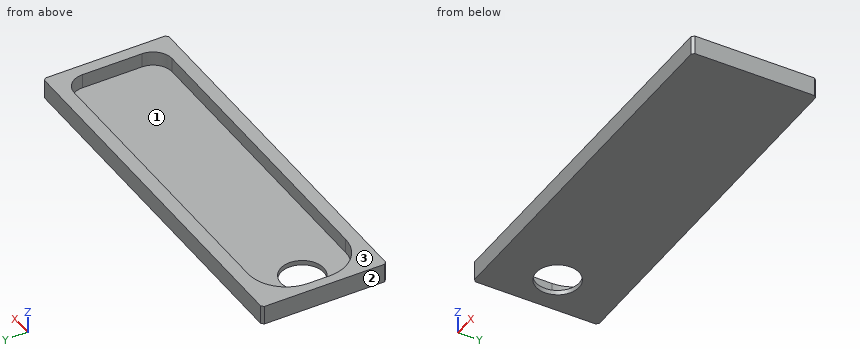
from build123d import *

# Parameters (mm, degrees)
F1_DEPTH = 3
F0_R     = 4.5
F2_DEPTH = 1
F3_SIZE  = 0.5


with BuildPart() as f1:
    # F0 (on Top) → F1 (new body)
    with BuildSketch(Plane.XY):
        Polygon((71.2, 13.05), (-8, 13.1), (-8, -13.1), (71.2, -13.05), align=None)
        with BuildLine():
            ThreePointArc((-6, 2.25), (-3.6568542495, 7.9068542495), (2, 10.25))
            Line((2, 10.25), (64.7, 10.25))
            ThreePointArc((64.7, 10.25), (67.5284271247, 9.0784271247), (68.7, 6.25))
            Line((68.7, 6.25), (68.7, -6.25))
            ThreePointArc((68.7, -6.25), (67.5284271247, -9.0784271247), (64.7, -10.25))
            Line((64.7, -10.25), (2, -10.25))
            ThreePointArc((2, -10.25), (-3.6568542495, -7.9068542495), (-6, -2.25))
            Line((-6, -2.25), (-6, 2.25))
        make_face(mode=Mode.SUBTRACT)
    extrude(amount=F1_DEPTH)

    # F0 (on Top) → F2 (join)
    with BuildSketch(Plane.XY):
        Polygon((71.2, 13.05), (-8, 13.1), (-8, -13.1), (71.2, -13.05), align=None)
        with BuildLine():
            ThreePointArc((-6, 2.25), (-3.6568542495, 7.9068542495), (2, 10.25))
            Line((2, 10.25), (64.7, 10.25))
            ThreePointArc((64.7, 10.25), (67.5284271247, 9.0784271247), (68.7, 6.25))
            Line((68.7, 6.25), (68.7, -6.25))
            ThreePointArc((68.7, -6.25), (67.5284271247, -9.0784271247), (64.7, -10.25))
            Line((64.7, -10.25), (2, -10.25))
            ThreePointArc((2, -10.25), (-3.6568542495, -7.9068542495), (-6, -2.25))
            Line((-6, -2.25), (-6, 2.25))
        make_face(mode=Mode.SUBTRACT)
        with BuildLine():
            Line((64.7, 10.25), (2, 10.25))
            ThreePointArc((2, 10.25), (-3.6568542495, 7.9068542495), (-6, 2.25))
            Line((-6, 2.25), (-6, -2.25))
            ThreePointArc((-6, -2.25), (-3.6568542495, -7.9068542495), (2, -10.25))
            Line((2, -10.25), (64.7, -10.25))
            ThreePointArc((64.7, -10.25), (67.5284271247, -9.0784271247), (68.7, -6.25))
            Line((68.7, -6.25), (68.7, 6.25))
            ThreePointArc((68.7, 6.25), (67.5284271247, 9.0784271247), (64.7, 10.25))
        make_face()
        Circle(F0_R, mode=Mode.SUBTRACT)
    extrude(amount=-F2_DEPTH)

    # F3
    f3_edges = [f1.edges().sort_by_distance(p)[0] for p in [
        (-8, -13.1, 1),
        (-8, 13.1, 1),
        (71.2, -13.05, 1),
        (71.2, 13.05, 1),
    ]]
    chamfer(f3_edges, length=F3_SIZE)


solid = f1.part
Check sheet for the modelled part. Datum: model origin and axes. Units: mm. Face numbers are marked on the shaded views. Coordinates: 2 decimals unless noted, no trailing zeros. Write each loop counter-clockwise with the first axis right and the second up, starting at its lowest first coordinate (ties: lowest second). Pieces come first, ordered by that corner, then holes.
Item 1: Cross-section at D-D on y = -8.25. Record the boundary of the cut face in (x, z), then the cut area to 3 significant figures.
Numbers:
outline: (-8, -1) - (71.2, -1) - (71.2, 3) - (68.16, 3) - (68.16, 0) - (-3.29, 0) - (-3.29, 3) - (-8, 3) - close
area: 102 mm2
Item 2: Scan lines: probe 1 along Y at (x, z) = (58.5, 1.55); probe 2 along Y at (x, z) = (0, -0.7); probe 3 along X at (y, z) = (-1.25, 1.1). Record each from-to range of solid material in increasing order.
Numbers:
probe 1: y = -13.06 to -10.25, 10.25 to 13.06
probe 2: y = -13.09 to -4.5, 4.5 to 13.09
probe 3: x = -8 to -6, 68.7 to 71.2
Item 3: Mould release check, pull along X, two halves, no side actions. Record for the marked faces 1, 2 and 3: released by +X, released by -X, zero draft, split by the parting line, or undercut.
Numbers:
face 1: undercut
face 2: released by -X
face 3: zero draft
Item 4: Cross-section at C-C on x = 3. Record the boundary of the cut face in (y, z).
Numbers:
outline: (-13.09, -1) - (-3.35, -1) - (-3.35, 0) - (-10.25, 0) - (-10.25, 3) - (-13.09, 3) - close; (3.35, -1) - (13.09, -1) - (13.09, 3) - (10.25, 3) - (10.25, 0) - (3.35, 0) - close
Item 5: Cross-section at A-A on z = 1.45. Record the boundary of the cut face in (x, y).
Numbers:
outline: (-8, -12.6) - (-7.5, -13.1) - (70.7, -13.05) - (71.2, -12.55) - (71.2, 12.55) - (70.7, 13.05) - (-7.5, 13.1) - (-8, 12.6) - close; hole (-6, -2.25) arc R8 ccw to (2, -10.25) - (64.7, -10.25) arc R4 ccw to (68.7, -6.25) - (68.7, 6.25) arc R4 ccw to (64.7, 10.25) - (2, 10.25) arc R8 ccw to (-6, 2.25) - close
Item 6: Cross-section at B-B on y = 0. Record the boundary of the cut face in (x, z).
Numbers:
outline: (-8, -1) - (-4.5, -1) - (-4.5, 0) - (-6, 0) - (-6, 3) - (-8, 3) - close; (4.5, -1) - (71.2, -1) - (71.2, 3) - (68.7, 3) - (68.7, 0) - (4.5, 0) - close
Item 7: Depth check by flat-ended pin: pin 1 Ø1.5 at (x, z) = (32.5, 0.5) entering from -Y; pin 2 Ø6 at (x, y) = (42, -3) entering from +Z; pin 3 Ø1.5 at (x, z) = (34.5, 1) entering from +Y; pin 4 Ø14.5 at (x, y) = (0, 0) entering from +Z. Enter the tip coordinate at first touch or a pass-through.
Numbers:
pin 1: stops at y = -13.07
pin 2: stops at z = 0
pin 3: stops at y = 13.07
pin 4: stops at z = 3
